The listing builds one solid part. Answer for the finished solid, in the listing's coordinates (mm). A direction names the side the tool comes from. Round coordinates to 2 decimals unless told otherwise and drop trailing zeros. Write each loop counter-clockwise with the first axis right and the second up, starting at its lowest first coordinate (ties: lowest second). Pieces come first, ordered by that corner, then holes. Notation, with made-up numbers: (-38.5, 26) - (3.5, 26) arc R18 ccw to (3.5, 39) - close; hole circle Ø9 at (44.5, 25.5). An arc over 180 degrees is marked (long way). Answer as CSV lines item,"result". Start each with the question number.
Item 1: Straight lines are drawn through the part: line 1 along X through (y, z) = (508, 35); line 2 along Y through (x, z) = (-64, 31.5); line 3 along Y through (x, z) = (175, 36). For each, find the intervals that lie inside material, in ascending order. Write a range as [from, to].
Item 2: For a pull along X with two mould halves and no side action, classify faces 4 (the cylindrical face through (22.509, 499.408, 45.344)), 5 (the cylindrical face through (-39.685, 499.408, 51.596)), 6 (the flat face through (-260, -188, 80)), 7 (the flat face through (43.3, 514.618, 34.8)) as pulls with the +X half, pulls with the -X half, needs draft (parallel to the pull), parting line crosses it, or undercut.
Item 3: A cutting plane is placed at A-A on y = 216. Determine the outline of the cut face in (x, z).
Item 4: A cutting plane is placed at B-B on x = -103.5. State how many separate pieces and enclosed holes the cut face has, and give its area (3 significant figures).
Item 5: Flat-ended cylindrical pins translate along their axes: pin 1 (22 mm diameter, centred on y = -250, z = 82, fed in from -X); pin 2 (22 mm diameter, centred on x = 89.5, z = 78.5, fed in from +Y); pin 3 (10 mm diameter, centred on y = -196, z = 85, fed in from +X). Find the tip coordinate at first contact, or state that the pin passes through.
Item 6: Which of the six approach directions +Z, -Z, +X, -X, +Y, -Y give full straight-line access (tool end or side, diameter ignored) to faces 1 (the flat face through (-4, -275.194, 80)), 2 (the flat face through (-4, 20, 80)), 3 (the cylindrical face through (-3.685, 499.408, 51.596))?
```python
from build123d import *

# Parameters (mm, degrees)
SKETCH1_W           = 660
SKETCH1_H           = 400
BOSS_EXTRUDE1_DEPTH = 70
SKETCH2_W           = 70
SKETCH2_H           = 70
BOSS_EXTRUDE2_DEPTH = 140
SKETCH3_W           = 70
SKETCH3_H           = 60
BOSS_EXTRUDE3_DEPTH = 660
BOSS_EXTRUDE4_DEPTH = 70
SKETCH5_W           = 520
SKETCH5_H           = 55.194253578
BOSS_EXTRUDE5_DEPTH = 30
FILLET1_R           = 10
SKETCH6_R           = 17
SKETCH6_R_2         = 7
BOSS_EXTRUDE6_DEPTH = 30
SKETCH9_W           = 660.000414718
SKETCH9_H           = 140
BOSS_EXTRUDE7_DEPTH = 70
SKETCH10_W          = 520
SKETCH10_H          = 55.194253578
BOSS_EXTRUDE8_DEPTH = 30
FILLET2_R           = 10


with BuildPart() as part:
    # Sketch1 → Boss-Extrude1 (new body)
    with BuildSketch(Plane.XY):
        Rectangle(SKETCH1_W, SKETCH1_H)
    extrude(amount=BOSS_EXTRUDE1_DEPTH)

    # Sketch2 → Boss-Extrude2 (add)
    with BuildSketch(Plane(origin=(0, 200, 0), x_dir=(1, 0, 0), z_dir=(0, 1, 0))):
        with Locations((-295, -35)):
            Rectangle(SKETCH2_W, SKETCH2_H)
        with Locations((295, -35)):
            Rectangle(SKETCH2_W, SKETCH2_H)
    extrude(amount=BOSS_EXTRUDE2_DEPTH)

    # Sketch3 → Boss-Extrude3 (add)
    with BuildSketch(Plane(origin=(330, 0, 0), x_dir=(0, 0, -1), z_dir=(1, 0, 0))):
        with Locations((-35, 310)):
            Rectangle(SKETCH3_W, SKETCH3_H)
    extrude(amount=-BOSS_EXTRUDE3_DEPTH)

    # Sketch4 → Boss-Extrude4 (add)
    with BuildSketch(Plane.XY.offset(70)):
        with BuildLine():
            Line((-186.732097713, 484.618446846), (186.732097713, 484.618446846))
            ThreePointArc((186.732097713, 484.618446846), (288.516412558, 442.178022701), (330, 340))
            Line((330, 340), (-330, 340))
            ThreePointArc((-330, 340), (-288.516412558, 442.178022701), (-186.732097713, 484.618446846))
        make_face()
        with BuildLine():
            Line((-131.145584022, 414.4805226), (131.145584022, 414.4805226))
            ThreePointArc((131.145584022, 414.4805226), (153.253905114, 392.372201507), (131.145584022, 370.263880415))
            Line((131.145584022, 370.263880415), (-131.145584022, 370.263880415))
            ThreePointArc((-131.145584022, 370.263880415), (-153.253905114, 392.372201507), (-131.145584022, 414.4805226))
        make_face(mode=Mode.SUBTRACT)
    extrude(amount=-BOSS_EXTRUDE4_DEPTH)

    # Sketch5 → Boss-Extrude5 (add)
    with BuildSketch(Plane.XY.offset(70)):
        with Locations((0, 172.402873211)):
            Rectangle(SKETCH5_W, SKETCH5_H)
        with Locations((0, 112.402873211)):
            Rectangle(SKETCH5_W, SKETCH5_H)
        with Locations((0, 52.402873211)):
            Rectangle(SKETCH5_W, SKETCH5_H)
        with Locations((0, -7.597126789)):
            Rectangle(SKETCH5_W, SKETCH5_H)
        with Locations((0, -67.597126789)):
            Rectangle(SKETCH5_W, SKETCH5_H)
        with Locations((0, -127.597126789)):
            Rectangle(SKETCH5_W, SKETCH5_H)
    extrude(amount=BOSS_EXTRUDE5_DEPTH)

    # Fillet1
    fillet1_edges = [part.edges().sort_by_distance(p)[0] for p in [
        (0, 140, 100),
        (-260, 112.402873211, 100),
        (0, 84.805746422, 100),
        (260, 112.402873211, 100),
        (0, 80, 100),
        (-260, 52.402873211, 100),
        (0, 24.805746422, 100),
        (260, 52.402873211, 100),
        (0, 20, 100),
        (-260, -7.597126789, 100),
        (0, -35.194253578, 100),
        (260, -7.597126789, 100),
        (0, -40, 100),
        (-260, -67.597126789, 100),
        (0, -95.194253578, 100),
        (260, -67.597126789, 100),
        (0, -100, 100),
        (-260, -127.597126789, 100),
        (0, -155.194253578, 100),
        (260, -127.597126789, 100),
        (-260, 172.402873211, 100),
        (0, 144.805746422, 100),
        (260, 172.402873211, 100),
        (0, 200, 100),
    ]]
    fillet(fillet1_edges, radius=FILLET1_R)

    # Sketch6 → Boss-Extrude6 (add)
    with BuildSketch(Plane(origin=(0, 484.618446846, 0), x_dir=(1, 0, 0), z_dir=(0, 1, 0))):
        with Locations((-36, -35)):
            Circle(SKETCH6_R)
        with Locations((-36, -35)):
            Circle(SKETCH6_R_2, mode=Mode.SUBTRACT)
        with Locations((0, -35)):
            Circle(SKETCH6_R)
        with Locations((0, -35)):
            Circle(SKETCH6_R_2, mode=Mode.SUBTRACT)
        with Locations((36, -35)):
            Circle(SKETCH6_R)
        with Locations((36, -35)):
            Circle(SKETCH6_R_2, mode=Mode.SUBTRACT)
    extrude(amount=BOSS_EXTRUDE6_DEPTH)

    # Sketch9 → Boss-Extrude7 (add)
    with BuildSketch(Plane.XY.offset(70)):
        with Locations((0.000207359, -270)):
            Rectangle(SKETCH9_W, SKETCH9_H)
    extrude(amount=-BOSS_EXTRUDE7_DEPTH)

    # Sketch10 → Boss-Extrude8 (add)
    with BuildSketch(Plane.XY.offset(70)):
        with Locations((0, -187.597126789)):
            Rectangle(SKETCH10_W, SKETCH10_H)
        with Locations((0, -127.597126789)):
            Rectangle(SKETCH10_W, SKETCH10_H)
        with Locations((0, -247.597126789)):
            Rectangle(SKETCH10_W, SKETCH10_H)
    extrude(amount=BOSS_EXTRUDE8_DEPTH)

    # Fillet2
    fillet2_edges = [part.edges().sort_by_distance(p)[0] for p in [
        (-260, -127.597126789, 100),
        (0, -155.194253578, 100),
        (260, -127.597126789, 100),
        (0, -100, 100),
        (-260, -187.597126789, 100),
        (0, -215.194253578, 100),
        (260, -187.597126789, 100),
        (0, -160, 100),
        (-260, -247.597126789, 100),
        (0, -275.194253578, 100),
        (260, -247.597126789, 100),
        (0, -220, 100),
    ]]
    fillet(fillet2_edges, radius=FILLET2_R)


solid = part.part
```
Geometry says:
1,line 1,"x = [-53, -43], [-29, -19], [-17, -7], [7, 17], [19, 29], [43, 53]"
1,line 2,"y = [-340, 200], [280, 370.26], [414.48, 484.62]"
1,line 3,"y = [-340, 200], [280, 484.62]"
2,face 4,"undercut"
2,face 5,"undercut"
2,face 6,"pulls with the -X half"
2,face 7,"needs draft"
3,outline,"(-330, 0) - (-260, 0) - (-260, 70) - (-330, 70) - close; (260, 0) - (330, 0) - (330, 70) - (260, 70) - close"
4,separate pieces,"3"
4,enclosed holes,"0"
4,area,"61,900 mm^2"
5,pin 1,"stops at x = -260"
5,pin 2,"stops at y = 484.62"
5,pin 3,"stops at x = 260"
6,face 1,"+Z, +X, -X, -Y"
6,face 2,"+Z, +X, -X"
6,face 3,"+Y"
